```python
from build123d import *

# Parameters (mm, degrees)
SKETCH_1_W          = 70
SKETCH_1_H          = 100
EXTRUDE_1_DEPTH     = 40
SKETCH_3_W          = 20
SKETCH_3_H          = 20
CUT_EXTRUDE_1_DEPTH = 40
SKETCH_5_W          = 20
SKETCH_5_H          = 30
SKETCH_5_H_2        = 29.917444877
CUT_EXTRUDE_4_DEPTH = 40
SKETCH_13_W         = 40
SKETCH_13_H         = 16
CUT_EXTRUDE_5_DEPTH = 40
SKETCH_15_W         = 20
SKETCH_15_H         = 40
CUT_EXTRUDE_6_DEPTH = 40


with BuildPart() as part:
    # 草图1 → 凸台-拉伸1 (new body)
    with BuildSketch(Plane(origin=(0, 0, 0), x_dir=(1, 0, 0), z_dir=(0, 1, 0))):
        Rectangle(SKETCH_1_W, SKETCH_1_H)
    extrude(amount=EXTRUDE_1_DEPTH)

    # 草图3 → 切除-拉伸1 (cut)
    with BuildSketch(Plane.XZ):
        with Locations((-25, -32.719295767)):
            Rectangle(SKETCH_3_W, SKETCH_3_H)
        with Locations((25.007645878, -32.353993134)):
            Rectangle(SKETCH_3_W, SKETCH_3_H)
    extrude(amount=-CUT_EXTRUDE_1_DEPTH, mode=Mode.SUBTRACT)

    # 草图5 → 切除-拉伸4 (cut)
    with BuildSketch(Plane(origin=(0, 40, 0), x_dir=(1, 0, 0), z_dir=(0, 1, 0))):
        with Locations((15.536368654, -35)):
            Rectangle(SKETCH_5_W, SKETCH_5_H)
        with Locations((-14.909129338, -35.083562285)):
            Rectangle(SKETCH_5_W, SKETCH_5_H_2)
    extrude(amount=-CUT_EXTRUDE_4_DEPTH, mode=Mode.SUBTRACT)

    # 草图13 → 切除-拉伸5 (cut)
    with BuildSketch(Plane(origin=(0, 40, 0), x_dir=(1, 0, 0), z_dir=(0, 1, 0))):
        Rectangle(SKETCH_13_W, SKETCH_13_H)
    extrude(amount=-CUT_EXTRUDE_5_DEPTH, mode=Mode.SUBTRACT)

    # 草图15 → 切除-拉伸6 (cut)
    with BuildSketch(Plane(origin=(0, 40, 0), x_dir=(1, 0, 0), z_dir=(0, 1, 0))):
        with Locations((-0.091013634, 31.465991837)):
            Rectangle(SKETCH_15_W, SKETCH_15_H)
    extrude(amount=-CUT_EXTRUDE_6_DEPTH, mode=Mode.SUBTRACT)


solid = part.part
```
The listing builds one solid part. Answer for the finished solid, in the listing's coordinates (mm). A direction names the side the tool comes from. Give positions to 0.01 mm unless a question says otherwise; leave off trailing zeros. Order: outer loops, then holes, each group sorted by start corner. A loop starts at its lowest first (then second) coordinate and runs counter-clockwise, first axis right, second up. Notation, with made-up numbers: (19.25, 7) - (48.25, 7) arc R21 cw to (48.25, 18) - close; hole circle Ø7 at (32, 71). An arc over 180 degrees is marked (long way). Use one line per item in the form item = value. Start each with the question number.
(1) The mould has two halves that part along X. Classify faces 1 (the flat face through (-25, 20, -22.719)), 2 (the flat face through (-24.909, 20, 35)), 3 (the flat face through (-35, 20, 14)): released by +X, released by -X, zero draft, split by the parting line, or undercut.
(2) For faces 4 (the flat face through (15.008, 20, -32)), 5 (the flat face through (0, 20, -8)), 6 (the flat face through (-25, 20, -42.719)), 7 (the flat face through (-15, 20, 20.125)), 8 (the flat face through (9.909, 20, -30)), determine the directions among +Z, -Z, +X, -X, +Y, -Y from which every point of the face is accessible in a straight line to the end or side of a thin tool.
(3) A cutting plane is placed at A-A, the plane z = -17. Write down the section's boundary in (x, y).
(4) A cutting plane is placed at C-C, the plane x = -9. Write down the section's boundary in (y, z), then the cut area to 3 significant figures.
(5) A cutting plane is placed at B-B, the plane x = -17. Write down the section's boundary in (y, z), then the cut area to 3 significant figures.
(6) Flat-ended cylindrical pins translate along their axes: pin 1 Ø1.5 at (y, z) = (21.5, -39) entering from +X; pin 2 Ø4 at (x, y) = (-15.5, 22.5) entering from +Z; pin 3 Ø10 at (y, z) = (14, -34) entering from -X; pin 4 Ø16 at (x, y) = (24.5, 17) entering from +Z. Find the tip coordinate at first contact, or state that the pin passes through.
(7) Consider line 1 (Z direction, x = 18, y = 36); line 2 (X direction, y = 20, z = 45); line 3 (Z direction, x = -2.5, y = 36). Determine where each line is inside the solid, lowest interval first. Write a range as from..to.
(8) A cutting plane is placed at D-D, the plane z = 39. Write down the section's boundary in (x, y), then the cut area to 3 significant figures.
Ans:
q1.face_1 = zero draft
q1.face_2 = undercut
q1.face_3 = released by -X
q2.face_4 = +X, +Y, -Y
q2.face_5 = +Y, -Y
q2.face_6 = -X, +Y, -Y
q2.face_7 = +Z, +Y, -Y
q2.face_8 = -Z, +Y, -Y
q3.outline = (-35, 0) - (-10.09, 0) - (-10.09, 40) - (-35, 40) - close; (9.91, 0) - (35, 0) - (35, 40) - (9.91, 40) - close
q4.outline = (0, -11.47) - (40, -11.47) - (40, -8) - (0, -8) - close; (0, 8) - (40, 8) - (40, 20.12) - (0, 20.12) - close
q4.area = 624 mm^2
q5.outline = (0, -50) - (40, -50) - (40, -42.72) - (0, -42.72) - close; (0, -22.72) - (40, -22.72) - (40, -8) - (0, -8) - close; (0, 8) - (40, 8) - (40, 20.12) - (0, 20.12) - close
q5.area = 1,360 mm^2
q6.pin_1 = 15.01
q6.pin_2 = 20.12
q6.pin_3 = -15
q6.pin_4 = 50
q7.line_1 = -50..-42.35, -22.35..-8, 8..20
q7.line_2 = -35..-24.91, -4.91..5.54, 25.54..35
q7.line_3 = -11.47..-8, 8..50
q8.outline = (-35, 0) - (-24.91, 0) - (-24.91, 40) - (-35, 40) - close; (-4.91, 0) - (5.54, 0) - (5.54, 40) - (-4.91, 40) - close; (25.54, 0) - (35, 0) - (35, 40) - (25.54, 40) - close
q8.area = 1,200 mm^2
